Source: CAD feature listing. Evaluate the final solid. Frame: model axes, mm. A direction names the side the tool comes from. Give positions to 0.01 mm unless a question says otherwise; leave off trailing zeros. Loops run counter-clockwise (first coordinate to the right, second up) from the corner with the lowest first, then second, coordinate; pieces in that order, holes last. Notation, with made-up numbers: M -15.5,-6 L 32.5,-6 A14 cw 32.5,-1 Z; hole C 50,16.5 d2. An arc over 180 degrees is marked long. Write item = value, one per line.
from build123d import *


with BuildPart() as f1:
    # F0 (on Front) → F1 (revolve)
    with BuildSketch(Plane.XZ):
        with BuildLine():
            Line((54.165728, 0), (45, 0))
            Line((45, 0), (45, -3))
            Line((45, -3), (55.657942, -13.657942))
            Line((55.657942, -13.657942), (83.572924, -13.657942))
            ThreePointArc((83.572924, -13.657942), (84.949633, -14.207193), (85.570183, -15.55327))
            Line((85.570183, -15.55327), (86, -23.754671))
            Line((86, -23.754671), (90, -23.754671))
            Line((90, -23.754671), (89.480465, -13.841344))
            ThreePointArc((89.480465, -13.841344), (88.314374, -11.222261), (85.69529, -10.05617))
            Line((85.69529, -10.05617), (65.893709, -9.018413))
            ThreePointArc((65.893709, -9.018413), (63.274626, -7.852322), (62.108535, -5.233239))
            Line((62.108535, -5.233239), (60, 35))
            Line((60, 35), (56, 35))
            Line((56, 35), (54.165728, 0))
        make_face()
    revolve(axis=Axis((0, 0, -2), (0, 0, 1)))


solid = f1.part
1. Cut plane D-D, the plane z = 29. Return the cut outline in (x, y).
Derived:
outline = C 0,0 d120.63; hole C 0,0 d111.37
2. Cut plane C-C, the plane z = 11.5. Return the cut outline in (x, y).
Derived:
outline = C 0,0 d122.46; hole C 0,0 d109.54
3. Material intervals for probe 1 along Y at (x, z) = (-40.5, 29.5); probe 2 along X at (y, z) = (74.5, -19); probe 3 along Y at (x, z) = (-78, -17.5), sorted ascending. Write a range as from..to.
Derived:
probe_1 = -44.66..-38.26, 38.26..44.66
probe_2 = -50.05..-42.46, 42.46..50.05
probe_3 = -44.24..-35.44, 35.44..44.24
4. First-contact query: pin 1 Ø4 at (x, y) = (-69.5, 39) entering from +Z; pin 2 Ø10 at (x, z) = (-52.5, -3) entering from +Y; pin 3 Ø12 at (y, z) = (54, 18) entering from -X. Flat tips, straight axial feed; report the tip coordinate or a pass-through.
Derived:
pin_1 = -9.64
pin_2 = 39.85
pin_3 = -37.48
5. Cut plane A-A, the plane x = 0. Return the cut outline in (y, z), then the cut area to 3 significant figures.
Derived:
outline = M -90,-23.75 L -86,-23.75 L -85.57,-15.55 A2 cw -83.57,-13.66 L -55.66,-13.66 L -45,-3 L -45,0 L -54.17,0 L -56,35 L -60,35 L -62.11,-5.23 A4 cw -65.89,-9.02 L -85.7,-10.06 A4 ccw -89.48,-13.84 Z; M 45,-3 L 55.66,-13.66 L 83.57,-13.66 A2 cw 85.57,-15.55 L 86,-23.75 L 90,-23.75 L 89.48,-13.84 A4 ccw 85.7,-10.06 L 65.89,-9.02 A4 cw 62.11,-5.23 L 60,35 L 56,35 L 54.17,0 L 45,0 Z
area = 1,070 mm²
6. Pull-direction query (X, two-part tool) for faces 4 (the conical face through (-11.894, -53.562, 13.366)), 5 (the flat face through (40, -40, 35)), 6 (the conical face through (63.77, 20.08, -9.07)); classes: +X half, -X half, draft (parallel to the pull), parting line (faces both ways), or undercut.
Derived:
face_4 = undercut
face_5 = draft
face_6 = parting line
7. Reachability of faces 1 (the flat face through (-17, -55, -13.658)), 2 (the flat face through (-46, -73, -23.755)), 3 (the flat face through (-20.3, 40.4, 0)) from +Z, -Z, +X, -X, +Y, -Y: full face, straight path, thin tool, end or side. Return the list, or none.
Derived:
face_1 = -Z
face_2 = -Z, +X, -X, +Y, -Y
face_3 = +Z
